For this review, take the finished solid that the model builds, in its own axes (mm). Face numbers are marked on the shaded views. Give positions to 0.01 mm unless a question says otherwise; leave off trailing zeros. Order: outer loops, then holes, each group sorted by start corner. A loop starts at its lowest first (then second) coordinate and runs counter-clockwise, first axis right, second up. Notation, with made-up numbers: (-35.5, 0) -> (-11.5, 0) arc R19 ccw to (-11.5, 4) -> close; hole circle Ø3 at (73.25, 67). An arc over 180 degrees is marked (long way). Use CSV: the item, a comma, the result in double quotes. Start each with the question number.
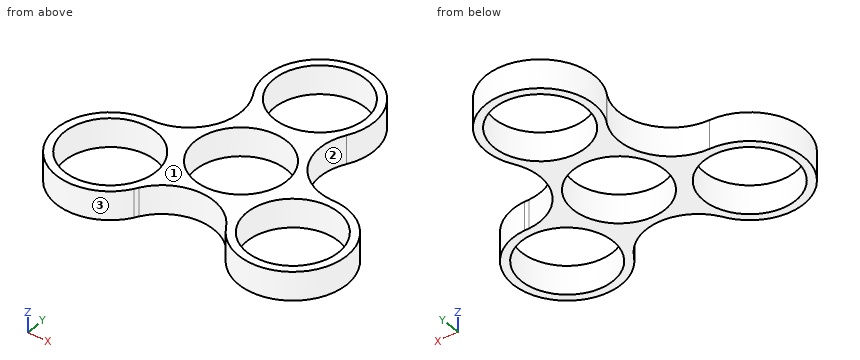
```python
from build123d import *

# Parameters (mm, degrees)
F0_R     = 11.2
F1_DEPTH = 7


with BuildPart() as f1:
    # F0 (on Top) → F1 (new body)
    with BuildSketch(Plane.XY):
        with BuildLine():
            ThreePointArc((21.845364, 0.267829), (11.320024, 6.836361), (11.431535, 19.242648))
            ThreePointArc((11.431535, 19.242648), (0.298709, 39.039268), (-11.71846, 19.766654))
            ThreePointArc((-11.71846, 19.766654), (-11.425584, 19.281984), (-11.154628, 18.784726))
            ThreePointArc((-11.154628, 18.784726), (-11.580474, 6.385248), (-22.38039, 0.278676))
            ThreePointArc((-22.38039, 0.278676), (-33.958352, -19.260944), (-11.259195, -20.031811))
            ThreePointArc((-11.259195, -20.031811), (-10.985896, -19.535837), (-10.690736, -19.052554))
            ThreePointArc((-10.690736, -19.052554), (0.26045, -13.221608), (10.948854, -19.521324))
            ThreePointArc((10.948854, -19.521324), (33.659643, -19.778324), (22.977655, 0.265157))
            ThreePointArc((22.977655, 0.265157), (22.41148, 0.253854), (21.845364, 0.267829))
        make_face()
        with Locations((-22.38039, -12.921324)):
            Circle(F0_R, mode=Mode.SUBTRACT)
        with Locations((22.38039, -12.921324)):
            Circle(F0_R, mode=Mode.SUBTRACT)
        Circle(F0_R, mode=Mode.SUBTRACT)
        with Locations((0, 25.842648)):
            Circle(F0_R, mode=Mode.SUBTRACT)
    extrude(amount=F1_DEPTH)


solid = f1.part
```
1. To check wall thickness, follow L1, parallel to X at y = -13, z = 0.5; L2, parallel to Y at x = 0, z = 5; L3, parallel to X at y = -22.5, z = 2.75. State the ranges of each line that lie inside material, in increasing order. Write a range as [from, to].
2. Clearance check with flat-ended pins moving along their axes: P1, Ø1.5, axis at y = 4, z = 5, coming from the +X side; P2, Ø3, axis at x = -25.5, z = 2, coming from the -Y side. State where each tip first meets the part, or that it passes through.
3. Consider section B-B (y = 9.5). State the section outline as (x, z) points, plus the area to 3 significant figures.
4. Consider section A-A (x = 0). State the section outline as (y, z) points, plus the area to 3 significant figures.
5. Consider section D-D (x = -18). State the section outline as (y, z) points, plus the area to 3 significant figures.
6. Consider section C-C (y = -9). State the section outline as (x, z) points, plus the area to 3 significant figures.
7. Draft analysis for pull direction Y (two halves, no side actions). For the marked faces 1, 2 and 3, state which applies: +Y half, -Y half, draft (parallel to the pull), parting line (faces both ways), or undercut.
Answer list:
1,L1,"[-35.58, -33.58], [-11.18, 11.18], [33.58, 35.58]"
1,L2,"[-13.22, -11.2], [11.2, 14.64], [37.04, 39.04]"
1,L3,"[-31.46, -28.18], [-16.58, -13.3], [13.3, 16.58], [28.18, 31.46]"
2,P1,"x = 14.25"
2,P2,"y = -26.02"
3,outline,"(-10.22, 0) -> (-5.93, 0) -> (-5.93, 7) -> (-10.22, 7) -> close; (5.93, 0) -> (10.23, 0) -> (10.23, 7) -> (5.93, 7) -> close"
3,area,"60.1 mm2"
4,outline,"(-13.22, 0) -> (-11.2, 0) -> (-11.2, 7) -> (-13.22, 7) -> close; (11.2, 0) -> (14.64, 0) -> (14.64, 7) -> (11.2, 7) -> close; (37.04, 0) -> (39.04, 0) -> (39.04, 7) -> (37.04, 7) -> close"
4,area,"52.2 mm2"
5,outline,"(-25.37, 0) -> (-23.23, 0) -> (-23.23, 7) -> (-25.37, 7) -> close; (-2.61, 0) -> (1.08, 0) -> (1.08, 7) -> (-2.61, 7) -> close"
5,area,"40.8 mm2"
6,outline,"(-34.98, 0) -> (-32.87, 0) -> (-32.87, 7) -> (-34.98, 7) -> close; (-11.89, 0) -> (-6.67, 0) -> (-6.67, 7) -> (-11.89, 7) -> close; (6.67, 0) -> (11.89, 0) -> (11.89, 7) -> (6.67, 7) -> close; (32.87, 0) -> (34.98, 0) -> (34.98, 7) -> (32.87, 7) -> close"
6,area,"103 mm2"
7,face 1,"draft"
7,face 2,"undercut"
7,face 3,"parting line"
